Autodesk Inventor part; units mm, degrees
ref_plane "YZ Plane" through (0, 0, 0) normal (1, 0, 0) x (0, 1, 0)
ref_plane "XZ Plane" through (0, 0, 0) normal (0, 1, 0) x (-1, 0, 0)
ref_plane "XY Plane" through (0, 0, 0) normal (0, 0, 1) x (1, 0, 0)
sketch "Sketch1" plane through (0, 0, 0) normal (0, 1, 0) x (-1, 0, 0)
  point P0 (0, 0)
sketch "Sketch2" plane through (0, 0, 0) normal (0, 1, 0) x (-1, 0, 0)
  line L0 (70, -12) -> (70, -66)
  line L1 (70, -66) -> (2, -66)
  line L2 (70, -12) -> (2, -12)
  line L3 (2, -66) -> (2, -12)
  point P0 (0, 0)
  point P1 (2, 0)
  dimension "d151" = 68
  dimension "d152" = 54
extrude "Extrusion1" add sketch "Sketch2" along normal blind 13
sketch "Sketch3" plane through (0, 13, 0) normal (0, 1, 0) x (1, 0, 0)
  point P0 (0, 0)
sketch "Sketch4" plane through (0, 13, 0) normal (0, 1, 0) x (1, 0, 0)
  line L0 (-2, 66) -> (-70, 66)
  line L1 (-30.4814, 66) -> (-28.4814, 66)
  line L2 (-28.4814, 66) -> (-28.4814, 64)
  line L3 (-70, 66) -> (-70, 12)
  line L4 (-70, 37.8423) -> (-70, 39.8423)
  line L5 (-70, 39.8423) -> (-68, 39.8423)
  line L6 (-68, 64) -> (-68, 14)
  line L7 (-68, 64) -> (-4, 64)
  line L8 (-68, 14) -> (-4, 14)
  line L9 (-4, 14) -> (-4, 64)
  line L10 (-70, 12) -> (-2, 12)
  line L11 (-2, 12) -> (-2, 66)
  point P0 (-2, 64)
  point P1 (-68, 12)
  dimension "d6" = 2
  dimension "d8" = 2
  dimension "d102" = 2
  dimension "d104" = 2
  dimension "d153" = 2
  dimension "d154" = 2
extrude "Extrusion2" cut sketch "Sketch4" against normal blind 12 contours L7 L9 L8 L6
sketch "Sketch10" plane through (0, 1, 0) normal (0, 1, 0) x (1, 0, 0)
  line L0 (-48, 14) -> (-48, 17)
  line L1 (-48, 14) -> (-63, 14)
  line L2 (-63, 14) -> (-63, 17)
  line L3 (-63, 17) -> (-48, 17)
  line L4 (-48, 17) -> (-48, 14)
  line L5 (-22, 64) -> (-7, 64)
  line L6 (-7, 64) -> (-7, 61)
  line L7 (-7, 61) -> (-22, 61)
  line L8 (-22, 61) -> (-22, 64)
  line L9 (-68, 64) -> (-4, 64)
  line L10 (-63, 14) -> (-48, 14)
  line L11 (-4, 14) -> (-68, 14)
  point P0 (-68, 2)
  point P1 (-2, 64)
  dimension "d55" = 3
  dimension "d56" = 15
  dimension "d60" = 15
  dimension "d108" = 3
  dimension "d155" = 0
extrude "Extrusion5" add sketch "Sketch10" along normal blind 6
sketch "Sketch12" plane through (0, 0, 0) normal (0, -1, 0) x (1, 0, 0)
  line L0 (0, 0) -> (0, -66)
  line L1 (-2, -12) -> (-2, -66)
  line L2 (-2, -66) -> (-70, -66)
  line L3 (-2, -66) -> (-70, -66)
  line L4 (-36, -66) -> (-36, -12)
  line L5 (-70, -66) -> (-70, -12)
  line L6 (-70, -66) -> (-70, -12)
  line L7 (-70, -39) -> (-2, -39)
  line L8 (-36, -39) -> (-36, -66)
  line L9 (-70, -66) -> (-36, -66)
  arc A0 (-56.4641, -41) -> (-56.4641, -37) centre (-53, -39) ccw
  line L10 (-53, -39) -> (-59.5, -39)
  arc A1 (-59.5, -37) -> (-59.5, -41) centre (-59.5, -39) ccw
  line L11 (-59.5, -41) -> (-56.4641, -41)
  line L12 (-59.5, -37) -> (-56.4641, -37)
  dimension "d158" = 8
  dimension "d159" = 6.5
  dimension "d160" = 4
extrude "Extrusion7" cut sketch "Sketch12" against normal blind 6 contours A0 L11 A1 L7 | L7 A1 L12 A0
sketch "Sketch13" plane through (0, 13, 0) normal (0, 1, 0) x (1, 0, 0)
  line L0 (-70, 66) -> (-70, 12)
  line L1 (-69, 65) -> (-69, 13)
  line L2 (-2, 66) -> (-70, 66)
  line L3 (-68, 64) -> (-4, 64)
  line L4 (-2, 64) -> (-2, 12)
  line L5 (-68, 14) -> (-68, 64)
  line L6 (-4, 14) -> (-68, 14)
  line L7 (-68, 14) -> (-4, 14)
  line L8 (-7, 64) -> (-4, 64)
  line L9 (-4, 14) -> (-4, 64)
  line L10 (-70, 12) -> (-2, 12)
  line L11 (-68, 13) -> (-69, 13)
  line L12 (-68, 13) -> (-3, 13)
  line L13 (-2, 12) -> (-2, 66)
  line L14 (-4, 13) -> (-3, 13)
  line L15 (-3, 13) -> (-3, 64)
  line L16 (-3, 64) -> (-3, 65)
  line L17 (-3, 65) -> (-69, 65)
  dimension "d96" = 1
  dimension "d99" = 1
extrude "Extrusion8" cut sketch "Sketch13" against normal blind 2 contours L17 L16 L15 L12 L11 L1 | L3 L9 L6 L5
sketch "Sketch15" plane through (-70, 0, -66) normal (-1, 0, 0) x (0, 0, 1)
  line L0 (62.4242, 8) -> (52.7396, 8)
  line L1 (0, 0) -> (66, 0)
  line L2 (0, 13) -> (54, 13)
  line L3 (0, 0) -> (0, 13)
  line L4 (18.77, 12) -> (27.77, 12)
  line L5 (27.77, 12) -> (27.77, 17)
  line L6 (27.77, 17) -> (18.77, 17)
  line L7 (18.77, 17) -> (18.77, 12)
  point P0 (66, 14)
  dimension "d118" = 8
  dimension "d140" = 27.77
  dimension "d141" = 9
  dimension "d143" = 5
  dimension "d150" = 4
extrude "Extrusion9" cut sketch "Sketch15" against normal blind 10
sketch "Sketch16" plane through (-2, 0, -66) normal (0, 0, -1) x (-1, 0, 0)
  line L0 (39.4, 13) -> (47.9, 13)
  line L1 (47.9, 13) -> (47.9, 8)
  line L2 (47.9, 8) -> (39.4, 8)
  line L3 (39.4, 8) -> (39.4, 13)
  line L4 (54.5, 13) -> (63, 13)
  line L5 (63, 13) -> (63, 8)
  line L6 (63, 8) -> (54.5, 8)
  line L7 (54.5, 8) -> (54.5, 13)
  line L8 (20, 7) -> (5, 7)
  line L9 (68, 0) -> (68, 13)
  point P0 (-2, 0)
  dimension "d127" = 8.5
  dimension "d128" = 8.5
  dimension "d131" = 28.6
  dimension "d132" = 13.5
  dimension "d148" = 5
  dimension "d149" = 6
extrude "Extrusion10" cut sketch "Sketch16" against normal blind 10
fillet "Fillet8" radius 3 1 edges at (-70, 6.5, -66)
sketch "Sketch17" plane through (0, 1, 0) normal (0, 1, 0) x (1, 0, 0)
  line L0 (-58.6569, 46) -> (-59.5, 46)
  arc A0 (-59.5, 46) -> (-59.5, 32) centre (-59.5, 39) ccw
  line L1 (-59.5, 32) -> (-58.6569, 32)
  arc A1 (-58.6569, 32) -> (-58.6569, 46) centre (-53, 39) ccw
  line L2 (-58.2915, 45) -> (-59.5, 45)
  arc A2 (-59.5, 45) -> (-59.5, 33) centre (-59.5, 39) ccw
  line L3 (-59.5, 33) -> (-58.2915, 33)
  arc A3 (-58.2915, 33) -> (-58.2915, 45) centre (-53, 39) ccw
  point P0 (0, 0)
  dimension "d165" = 1
extrude "Extrusion11" add sketch "Sketch17" along normal blind 5 contours A1 L1 A0 L0 | A3 L3 A2 L2
sketch "Sketch18" plane through (0, 6, 0) normal (0, 1, 0) x (1, 0, 0)
  arc A0 (-56.4641, 37) -> (-56.4641, 41) centre (-53, 39) ccw
  arc A1 (-58.7115, 32.0445) -> (-58.7115, 45.9555) centre (-53, 39) ccw
  arc A2 (-59.5, 41) -> (-59.5, 37) centre (-59.5, 39) ccw
  arc A3 (-58.7115, 45.9555) -> (-58.7115, 32.0445) centre (-59.5, 39) ccw
  arc A4 (-58.4038, 33.101) -> (-58.4038, 44.899) centre (-53, 39) ccw
  arc A5 (-58.4038, 44.899) -> (-58.4038, 33.101) centre (-59.5, 39) ccw
  point P0 (0, 0)
  dimension "d166" = 1
extrude "Extrusion12" cut sketch "Sketch18" against normal blind 5 contours A5 A4
sketch "Sketch19" plane through (0, 6, 0) normal (0, 1, 0) x (1, 0, 0)
  arc A0 (-59.5, 41) -> (-59.5, 37) centre (-59.5, 39) ccw
  arc A1 (-58.788, 45.9637) -> (-58.788, 32.0363) centre (-59.5, 39) ccw
  arc A2 (-56.4641, 37) -> (-56.4641, 41) centre (-53, 39) ccw
  arc A3 (-58.788, 32.0363) -> (-58.788, 45.9637) centre (-53, 39) ccw
  point P0 (0, 0)
extrude "Extrusion13" add sketch "Sketch19" against normal blind 1
properties part number "Shell 5 bottom"
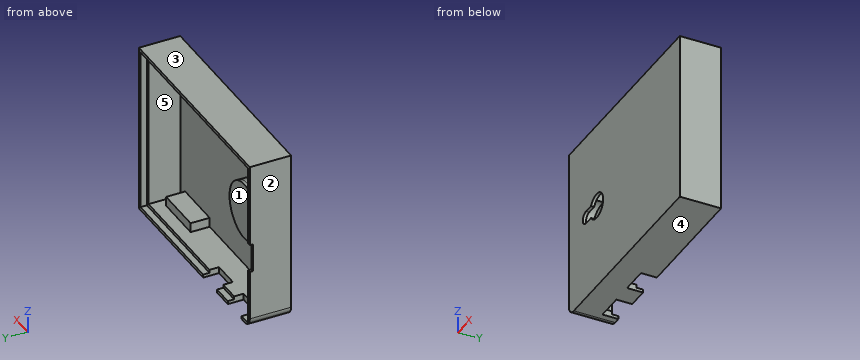
Geometry: final body of the model. Coordinates: model frame, mm. Face numbers are marked on the shaded views. A direction names the side the tool comes from. Coordinates: 2 decimals unless noted, no trailing zeros. Order: outer loops, then holes, each group sorted by start corner. A loop starts at its lowest first (then second) coordinate and runs counter-clockwise, first axis right, second up. Notation, with made-up numbers: M 11.25,16.25 L 37.25,16.25 A36 cw 37.25,51.25 Z; hole C 53,57 d3. An arc over 180 degrees is marked long. One line per question, with ' | ' between items. Start each with the question number.
Item 1: Cut plane A-A, the plane y = 4. Return the cut outline in (x, z).
Item 2: Draft query along Z for the marked faces 3, 4 and 5. Return one class per face: released by +Z, released by -Z, zero draft, split by the parting line, or undercut.
Item 3: Cut plane C-C, the plane z = -60. Return the cut outline in (x, y), then the cut area to 3 significant figures.
Item 4: Ray query, probe 1 along Z at (x, y) = (-53, 3.3); probe 2 along X at (y, z) = (3.3, -39); probe 3 along X at (y, z) = (1.75, -27.5). Return the intervals inside material, ascending. Write a range as [from, to].
Item 5: Set-up query: the marked faces 1 and 2. Return all of +Z, -Z, +X, -X, +Y, -Y with unobstructed straight access to the full face (end or side cutting, diameter ignored); none if empty.
Item 6: Pin query (flat end, axial travel): pin 1 Ø1.6 at (y, z) = (10, -64.5) entering from -X; pin 2 Ø0.9 at (x, z) = (-54.5, -15) entering from +Y; pin 3 Ø4 at (x, z) = (-10.5, -52.5) entering from +Y. Return the tip coordinate at first contact, or that it passes through.
Item 7: Cut plane B-B, the plane x = -38. Return the cut outline in (y, z), then the cut area to 3 significant figures.
A:
1) outline: M -70,-63 A3 ccw -67,-66 L -2,-66 L -2,-12 L -70,-12 Z; M -59.5,-46 L -58.66,-46 A9 ccw long -58.66,-32 L -59.5,-32 A7 ccw Z; hole M -68,-64 L -22,-64 L -22,-61 L -7,-61 L -7,-64 L -4,-64 L -4,-14 L -48,-14 L -48,-17 L -63,-17 L -63,-14 L -68,-14 Z; hole M -58.4,-44.9 A8 ccw long -58.4,-33.1 A6 ccw long Z
2) face 3: released by +Z | face 4: released by -Z | face 5: undercut
3) outline: M -70,0 L -2,0 L -2,13 L -3,13 L -3,11 L -4,11 L -4,1 L -68,1 L -68,11 L -69,11 L -69,13 L -70,13 Z | area: 112 mm2
4) probe 1: z = [-66, -64], [-48, -47], [-31, -30], [-17, -12] | probe 2: x = [-70, -68], [-66.5, -65.5], [-45, -44], [-4, -2] | probe 3: x = [-70, -68], [-4, -2]
5) face 1: +Y | face 2: +Z, -Z, -X, +Y, -Y
6) pin 1: stops at x = -69.92 | pin 2: stops at y = 7 | pin 3: stops at y = 1
7) outline: M 0,-66 L 13,-66 L 13,-65 L 11,-65 L 11,-64 L 1,-64 L 1,-14 L 11,-14 L 11,-13 L 13,-13 L 13,-12 L 0,-12 Z | area: 98.0 mm2
